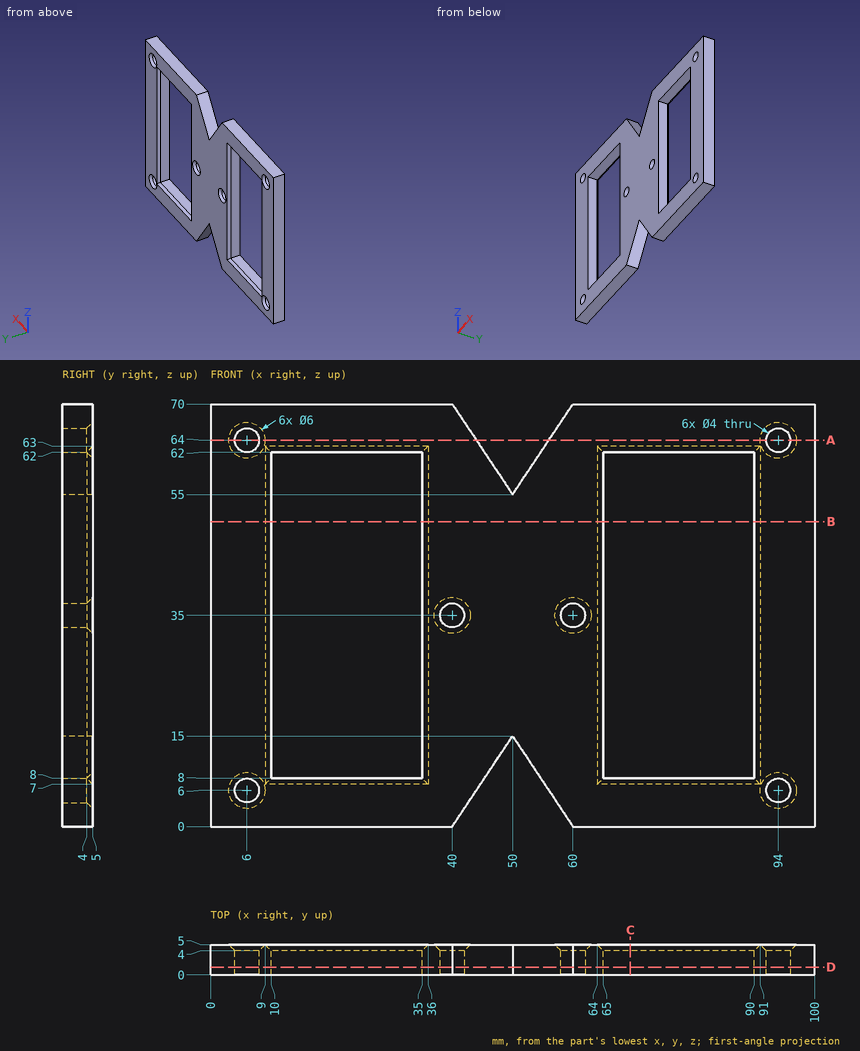
Verification items for this drawing (mm, ordinates from the low corner). Coordinates: 2 decimals unless noted, no trailing zeros. Write each loop counter-clockwise with the first axis right and the second up, starting at its lowest first coordinate (ties: lowest second). Pieces come first, ordered by that corner, then holes. Notation, with made-up numbers: (2, 79) -> (26, 79) arc R25 ccw to (26, 117) -> close; hole circle Ø3 at (-27, -24). An arc over 180 degrees is marked (long way). Use CSV: the item, a comma, the result in double quotes. Start each with the question number.
Item 1: Thickness scan on line 1 (X direction, y = 2, z = 35); line 2 (Z direction, x = 94, y = 2.85); line 3 (X direction, y = 3.6, z = 48). Record the ranges inside material, lowest first.
Item 2: Cross-section at D-D, the plane y = 1.3. State how many separate pieces and enclosed holes the cut face has, plus the area to 3 significant figures.
Item 3: Depth check by flat-ended pin: pin 1 Ø6.5 at (x, z) = (94, 6) entering from +Y; pin 2 Ø5 at (x, z) = (40, 35) entering from +Y; pin 3 Ø1 at (x, y) = (49, 1.5) entering from -Z. Enter the tip coordinate at first touch or a pass-through.
Item 4: Cross-section at C-C, the plane x = 69.5. Record the cut outline in (y, z).
Item 5: Cross-section at B-B, the plane z = 50.5. Record the cut outline in (x, y), plus the area to 3 significant figures.
Item 6: Cross-section at A-A, the plane z = 64. Record the cut outline in (x, y), plus the area to 3 significant figures.
Answers:
1,line 1,"0 to 10, 35 to 38, 42 to 58, 62 to 65, 90 to 100"
1,line 2,"0 to 4, 8 to 62, 66 to 70"
1,line 3,"0 to 10, 35 to 65, 90 to 100"
2,separate pieces,"1"
2,enclosed holes,"8"
2,area,"3,920 mm^2"
3,pin 1,"y = 5"
3,pin 2,"y = 4.5"
3,pin 3,"z = 12.75"
4,outline,"(0, 0) -> (5, 0) -> (5, 7) -> (4, 8) -> (0, 8) -> close; (0, 62) -> (4, 62) -> (5, 63) -> (5, 70) -> (0, 70) -> close"
5,outline,"(0, 0) -> (10, 0) -> (10, 4) -> (9, 5) -> (0, 5) -> close; (35, 0) -> (65, 0) -> (65, 4) -> (64, 5) -> (36, 5) -> (35, 4) -> close; (90, 0) -> (100, 0) -> (100, 5) -> (91, 5) -> (90, 4) -> close"
5,area,"248 mm^2"
6,outline,"(0, 0) -> (4, 0) -> (4, 4) -> (3, 5) -> (0, 5) -> close; (8, 0) -> (44, 0) -> (44, 5) -> (9, 5) -> (8, 4) -> close; (56, 0) -> (92, 0) -> (92, 4) -> (91, 5) -> (56, 5) -> close; (96, 0) -> (100, 0) -> (100, 5) -> (97, 5) -> (96, 4) -> close"
6,area,"398 mm^2"
